Geometry check sheet. Reference: the model listing, model coordinates, mm. A direction names the side the tool comes from. Round coordinates to 2 decimals unless told otherwise and drop trailing zeros. Write each loop counter-clockwise with the first axis right and the second up, starting at its lowest first coordinate (ties: lowest second). Pieces come first, ordered by that corner, then holes.
Item 1: Cross-section at B-B (z = -25.5). Enter the section's corners in (x, y).
Item 2: Access from +Z, -Z, +X, -X, +Y, -Y to the whole of each face (thin tool, end or side, straight path). Record for faces 1 (the face through (15, -195, -17)), 2 (the face through (-12, -99, -46)), 3 (the face through (-9, -99, -43)), 4 (the face through (3, -99, -61)).
Item 3: Cross-section at C-C (z = -43.5). Enter the section's corners in (x, y), then the cut area to 3 significant figures.
Item 4: Cross-section at A-A (x = 0). Enter the section's corners in (y, z).
Item 5: Depth check by flat-ended pin: P1, Ø10, axis at x = 20.5, y = -31.5, coming from the +Z side; P2, Ø24, axis at y = -98.5, z = -45.5, coming from the -X side; P3, Ø11, axis at y = -3, z = -10, coming from the +X side. Enter the tip coordinate at first touch or a pass-through.
Item 6: Draft check along Y on faces 5 (the face through (6, -99, -58)), 6 (the face through (12.15, -194.93, 11.99)). Enter one of: pulls with the +Y half, pulls with the -Y half, needs draft (parallel to the pull), parting line crosses it, or undercut.
Item 7: Scan lines: probe 1 along Y at (x, z) = (-10, 8.5); probe 2 along Z at (x, y) = (0, -4.25); probe 3 along X at (y, z) = (-68.5, -45). Record each from-to range of solid material in increasing order.
Item 8: Cross-section at D-D (x = 23). Enter the section's corners in (y, z).
from build123d import *

# Parameters (mm, degrees)
F0_R     = 9
F1_DEPTH = 10
F7_DEPTH = 180
F8_R     = 9
F9_DEPTH = 10


# Not quite as in the source:
# - a feature of the source that left no trace in its solid (it failed there, or was rolled back) is left out


with BuildPart() as f1:
    # F0 (on Front) → F1 (new body)
    with BuildSketch(Plane.XZ):
        with BuildLine():
            Line((5, 15), (-5, 15))
            ThreePointArc((-5, 15), (-12.0710678119, 12.0710678119), (-15, 5))
            Line((-15, 5), (-15, -54))
            ThreePointArc((-15, -54), (-12.0710678119, -61.0710678119), (-5, -64))
            Line((-5, -64), (44.0328441188, -64))
            Line((44.0328441188, -64), (44.0328441188, -20))
            Line((44.0328441188, -20), (19.9575467156, -40.731087613))
            ThreePointArc((19.9575467156, -40.731087613), (16.7495281184, -41.1847233597), (15, -38.4577616671))
            Line((15, -38.4577616671), (15, 5))
            ThreePointArc((15, 5), (12.0710678119, 12.0710678119), (5, 15))
        make_face()
        Circle(F0_R, mode=Mode.SUBTRACT)
    extrude(amount=F1_DEPTH)

    # F6 (on face) → F7 (join)
    with BuildSketch(Plane.XZ.offset(10)):
        with BuildLine():
            Line((-12, -61), (18, -61))
            Line((18, -61), (18, -60.5))
            ThreePointArc((18, -60.5), (17.267766953, -58.732233047), (15.5, -58))
            Line((15.5, -58), (-4, -58))
            ThreePointArc((-4, -58), (-7.5355339059, -56.5355339059), (-9, -53))
            Line((-9, -53), (-9, -33.5))
            ThreePointArc((-9, -33.5), (-9.732233047, -31.732233047), (-11.5, -31))
            Line((-11.5, -31), (-12, -31))
            Line((-12, -31), (-12, -61))
        make_face()
    extrude(amount=F7_DEPTH)

    # F8 (on face) → F9 (join)
    with BuildSketch(Plane.XZ.offset(190)):
        with BuildLine():
            Line((5, 15), (-5, 15))
            ThreePointArc((-5, 15), (-12.0710678119, 12.0710678119), (-15, 5))
            Line((-15, 5), (-15, -54))
            ThreePointArc((-15, -54), (-12.0710678119, -61.0710678119), (-5, -64))
            Line((-5, -64), (44.0328441188, -64))
            Line((44.0328441188, -64), (44.0328441188, -20))
            Line((44.0328441188, -20), (19.9575467156, -40.731087613))
            ThreePointArc((19.9575467156, -40.731087613), (16.7495281184, -41.1847233597), (15, -38.4577616671))
            Line((15, -38.4577616671), (15, 5))
            ThreePointArc((15, 5), (12.0710678119, 12.0710678119), (5, 15))
        make_face()
        Circle(F8_R, mode=Mode.SUBTRACT)
    extrude(amount=F9_DEPTH)


solid = f1.part
Resolved:
1. outline: (-15, -200) - (15, -200) - (15, -190) - (-15, -190) - close; (-15, -10) - (15, -10) - (15, 0) - (-15, 0) - close; (37.65, -200) - (44.03, -200) - (44.03, -190) - (37.65, -190) - close; (37.65, -10) - (44.03, -10) - (44.03, 0) - (37.65, 0) - close
2. face 1: +Z, +Y, -Y
2. face 2: +Z, -Z, -X
2. face 3: +Z, +X
2. face 4: -Z, +X, -X
3. outline: (-15, -200) - (44.03, -200) - (44.03, -190) - (-9, -190) - (-9, -10) - (44.03, -10) - (44.03, 0) - (-15, 0) - (-15, -10) - (-12, -10) - (-12, -190) - (-15, -190) - close
3. area: 1,720 mm2
4. outline: (-200, -64) - (-190, -64) - (-190, -61) - (-10, -61) - (-10, -64) - (0, -64) - (0, -9) - (-10, -9) - (-10, -58) - (-190, -58) - (-190, -9) - (-200, -9) - close; (-200, 9) - (-190, 9) - (-190, 15) - (-200, 15) - close; (-10, 9) - (0, 9) - (0, 15) - (-10, 15) - close
5. P1: stops at z = -58
5. P2: stops at x = -12
5. P3: stops at x = 15
6. face 5: undercut
6. face 6: needs draft
7. probe 1: y = -200 to -190, -10 to 0
7. probe 2: z = -64 to -9, 9 to 15
7. probe 3: x = -12 to -9
8. outline: (-200, -64) - (-190, -64) - (-190, -38.11) - (-200, -38.11) - close; (-10, -64) - (0, -64) - (0, -38.11) - (-10, -38.11) - close
